```python
from build123d import *

# Parameters (mm, degrees)
BOSS_EXTRUDE1_DEPTH     = 15
CUT_EXTRUDE1_DEPTH      = 25.488909851
CUT_EXTRUDE1_DEPTH_BACK = 25.488909851


with BuildPart() as part:
    # Sketch1 → Boss-Extrude1 (new body)
    with BuildSketch(Plane(origin=(0, 0, 0), x_dir=(1, 0, 0), z_dir=(0, 1, 0))):
        Polygon((-10.767691547, 0), (-10.767691547, -10), (14.780280975, -12.5), (14.780280975, -5), (11.780280975, -5), (11.780280975, -9.192105414), (-7.767691547, -7.279236153), (-7.767691547, 0), (-7.767691547, 7.279236153), (11.780280975, 9.192105414), (11.780280975, 5), (14.780280975, 5), (14.780280975, 12.5), (-10.767691547, 10), align=None)
    extrude(amount=BOSS_EXTRUDE1_DEPTH)

    # Sketch2 → Cut-Extrude1 (cut, two sides: drawn at the far end of the back side and taken through both)
    with BuildSketch(Plane.XY.offset(-CUT_EXTRUDE1_DEPTH_BACK)):
        Polygon((14.780280975, 15), (14.780280975, 5.495203142), (-10.767691547, 10), (-10.767691547, 15), align=None)
    extrude(amount=CUT_EXTRUDE1_DEPTH + CUT_EXTRUDE1_DEPTH_BACK, mode=Mode.SUBTRACT)


solid = part.part
```
Source: CAD feature listing. Evaluate the final solid. Frame: model axes, mm. A direction names the side the tool comes from. Give positions to 0.01 mm unless a question says otherwise; leave off trailing zeros. Loops run counter-clockwise (first coordinate to the right, second up) from the corner with the lowest first, then second, coordinate; pieces in that order, holes last. Notation, with made-up numbers: (31.5, 57.25) - (78.5, 57.25) arc R17 ccw to (78.5, 74.25) - close; hole circle Ø2 at (39.5, 8). An arc over 180 degrees is marked (long way). Use CSV: the item, a comma, the result in double quotes.
1) Cut plane B-B (x = 0). Output: boundary loops of the cut face in (y, z), and give its area (3 significant figures).
Worked out:
outline,"(0, -11.05) - (8.1, -11.05) - (8.1, -8.04) - (0, -8.04) - close; (0, 8.04) - (8.1, 8.04) - (8.1, 11.05) - (0, 11.05) - close"
area,"48.8 mm^2"
2) Cut plane D-D (z = 2.25). Output: boundary loops of the cut face in (x, y).
Worked out:
outline,"(-10.77, 0) - (-7.77, 0) - (-7.77, 9.47) - (-10.77, 10) - close"
3) Cut plane A-A (z = -6.5). Output: boundary loops of the cut face in (x, y).
Worked out:
outline,"(-10.77, 0) - (-7.77, 0) - (-7.77, 9.47) - (-10.77, 10) - close; (11.78, 0) - (14.78, 0) - (14.78, 5.5) - (11.78, 6.02) - close"
4) Cut plane C-C (y = 4.5). Output: boundary loops of the cut face in (x, z).
Worked out:
outline,"(-10.77, -10) - (14.78, -12.5) - (14.78, -5) - (11.78, -5) - (11.78, -9.19) - (-7.77, -7.28) - (-7.77, 7.28) - (11.78, 9.19) - (11.78, 5) - (14.78, 5) - (14.78, 12.5) - (-10.77, 10) - close"
5) Pin query (flat end, axial travel): P1, Ø1.5, axis at y = 9, z = -3, coming from the +X side; P2, Ø0.9, axis at x = 14, y = 4, coming from the +Z side; P3, Ø2, axis at x = 6.5, y = 3.5, coming from the -Z side. Return the tip coordinate at first contact, or that it passes through.
Worked out:
P1,"stops at x = -7.77"
P2,"stops at z = 12.47"
P3,"stops at z = -11.79"
6) Mould query, pull axis Z, two halves, no side actions, for faces 4 (the flat face through (11.78, 3, 7)), 5 (the flat face through (14.78, 3, -9)), 6 (the flat face through (2.185, 3.819, -11.268)). Classes: +Z half, -Z half, draft (parallel to the pull), parting line (faces both ways), or undercut.
Worked out:
face 4,"undercut"
face 5,"draft"
face 6,"-Z half"
7) Set-up query: faces 1 (the flat face through (14.78, 3, 9)), 2 (the flat face through (13, 3, 5)), 3 (the flat face through (2.14, 3.62, 8.25)). Return all of +Z, -Z, +X, -X, +Y, -Y with unobstructed straight access to the full face (end or side cutting, diameter ignored); none if empty.
Worked out:
face 1,"+Z, -Z, +X, +Y, -Y"
face 2,"+X, +Y, -Y"
face 3,"+Y, -Y"
8) Line query: line 1 (X direction, y = 2, z = -5.5); line 2 (X direction, y = 7.5, z = -0.25); line 3 (Z direction, x = -6, y = 5.5). Output: solid intervals per line, ascending.
Worked out:
line 1,"x = -10.77 to -7.77, 11.78 to 14.78"
line 2,"x = -10.77 to -7.77"
line 3,"z = -10.47 to -7.45, 7.45 to 10.47"
